from build123d import *

# Parameters (mm, degrees)
F0_W         = 69
F0_H         = 5.7454954955
F1_DEPTH     = 2050
F2_W         = 10
F2_H         = 101.5
F3_DEPTH     = 7.5
F7_DEPTH     = 84
F10_DEPTH    = 90
F11_T1_DEPTH = 134.5
F12_T1_DEPTH = 139.5


# Not quite as in the source:
# - a fillet or chamfer that OpenCascade refuses, or shapes differently, is made with other operations: its cross-section is extruded or revolved along the edge and cut away or added


with BuildPart() as f1:
    # F0 (on Right) → F1 (new body)
    with BuildSketch(Plane.YZ):
        with BuildLine():
            ThreePointArc((-53.5, -33.75), (-51.1568542495, -39.4068542495), (-45.5, -41.75))
            Line((-45.5, -41.75), (0, -41.75))
            Line((0, -41.75), (0, -36.0045045045))
            Line((0, -36.0045045045), (-45.5, -36.0045045045))
            ThreePointArc((-45.5, -36.0045045045), (-48.3284271247, -34.8329316293), (-49.5, -32.0045045045))
            Line((-49.5, -32.0045045045), (-49.5, 32.0045045045))
            ThreePointArc((-49.5, 32.0045045045), (-48.3284271247, 34.8329316293), (-45.5, 36.0045045045))
            Line((-45.5, 36.0045045045), (0, 36.0045045045))
            Line((0, 36.0045045045), (0, 41.75))
            Line((0, 41.75), (-45.5, 41.75))
            ThreePointArc((-45.5, 41.75), (-51.1568542495, 39.4068542495), (-53.5, 33.75))
            Line((-53.5, 33.75), (-53.5, -33.75))
        make_face()
        with Locations((34.5, 38.8772522523)):
            Rectangle(F0_W, F0_H)
        with Locations((34.5, -38.8772522523)):
            Rectangle(F0_W, F0_H)
    extrude(amount=-F1_DEPTH)

    # F2 (on face) → F3 (join)
    with BuildSketch(Plane.XY.offset(41.75)):
        with Locations((-2039, 8.25)):
            Rectangle(F2_W, F2_H)
    extrude(amount=F3_DEPTH)

    # F5: F1 across plane


with BuildPart() as f1_1:
    add(f1.part)
    add(f1.part.mirror(Plane.YZ.offset(-1025)))

    # F6 (on face) → F7 (cut)
    with BuildSketch(Plane.XY.offset(41.75)):
        with BuildLine():
            Line((-2001, 39.5), (-2001, 0))
            Line((-2001, 0), (-2001, -37.5))
            ThreePointArc((-2001, -37.5), (-1998.6568542495, -43.1568542495), (-1993, -45.5))
            Line((-1993, -45.5), (-1925.5, -45.5))
            Line((-1925.5, -45.5), (-1925.5, -41.25))
            Line((-1925.5, -41.25), (-1984.9698543549, -41.25))
            Line((-1984.9698543549, -41.25), (-1992.75, -41.25))
            ThreePointArc((-1992.75, -41.25), (-1995.5784271247, -40.0784271247), (-1996.75, -37.25))
            Line((-1996.75, -37.25), (-1996.75, 0))
            Line((-1996.75, 0), (-1996.75, 39.25))
            ThreePointArc((-1996.75, 39.25), (-1995.5784271247, 42.0784271247), (-1992.75, 43.25))
            Line((-1992.75, 43.25), (-1925.5, 43.25))
            Line((-1925.5, 43.25), (-1925.5, 47.5))
            Line((-1925.5, 47.5), (-1993, 47.5))
            ThreePointArc((-1993, 47.5), (-1998.6568542495, 45.1568542495), (-2001, 39.5))
        make_face()
    extrude(amount=-F7_DEPTH, mode=Mode.SUBTRACT)

    # F8: F1 across plane


with BuildPart() as f1_2:
    add(f1_1.part)
    add(f1_1.part.mirror(Plane.YZ.offset(-1025)), mode=Mode.INTERSECT)

    # F9 (on face) → F10 (cut)
    with BuildSketch(Plane.XY.offset(41.75)):
        with BuildLine():
            ThreePointArc((-1024.0666470126, -40.75), (-1021.1231056256, -43.8556546004), (-1017, -45))
            Line((-1017, -45), (-950, -45))
            Line((-950, -45), (-950, -40.75))
            Line((-950, -40.75), (-1016.75, -40.75))
            ThreePointArc((-1016.75, -40.75), (-1019.5784271247, -39.5784271247), (-1020.75, -36.75))
            Line((-1020.75, -36.75), (-1020.75, 1.25))
            Line((-1020.75, 1.25), (-1020.75, 39.25))
            ThreePointArc((-1020.75, 39.25), (-1019.5784271247, 42.0784271247), (-1016.75, 43.25))
            Line((-1016.75, 43.25), (-950, 43.25))
            Line((-950, 43.25), (-950, 47.5))
            Line((-950, 47.5), (-1017, 47.5))
            ThreePointArc((-1017, 47.5), (-1021.1231056256, 46.3556546004), (-1024.0666470126, 43.25))
            Line((-1024.0666470126, 43.25), (-1025.9333529874, 43.25))
            ThreePointArc((-1025.9333529874, 43.25), (-1028.8768943744, 46.3556546004), (-1033, 47.5))
            Line((-1033, 47.5), (-1100, 47.5))
            Line((-1100, 47.5), (-1100, 43.25))
            Line((-1100, 43.25), (-1033.25, 43.25))
            ThreePointArc((-1033.25, 43.25), (-1030.4215728753, 42.0784271247), (-1029.25, 39.25))
            Line((-1029.25, 39.25), (-1029.25, 1.25))
            Line((-1029.25, 1.25), (-1029.25, -36.75))
            ThreePointArc((-1029.25, -36.75), (-1030.4215728753, -39.5784271247), (-1033.25, -40.75))
            Line((-1033.25, -40.75), (-1100, -40.75))
            Line((-1100, -40.75), (-1100, -45))
            Line((-1100, -45), (-1033, -45))
            ThreePointArc((-1033, -45), (-1028.8768943744, -43.8556546004), (-1025.9333529874, -40.75))
            Line((-1025.9333529874, -40.75), (-1024.0666470126, -40.75))
        make_face()
    extrude(amount=-F10_DEPTH, mode=Mode.SUBTRACT)

    # F11: fillet of radius 4 on 1 edges, made by hand

    # F11_s2 → F11_t1 (cut)
    with BuildSketch(Plane.XZ.offset(-79)):
        with BuildLine():
            ThreePointArc((-2046, -41.75), (-2048.8284271247, -40.5784271247), (-2050, -37.75))
            Line((-2050, -37.75), (-2050, -41.75))
            Line((-2050, -41.75), (-2046, -41.75))
        make_face()
    extrude(amount=F11_T1_DEPTH, mode=Mode.SUBTRACT)

    # F12: fillet of radius 5 on 1 edges, made by hand

    # F12_s2 → F12_t1 (cut)
    with BuildSketch(Plane.XZ.offset(-81.5)):
        with BuildLine():
            ThreePointArc((0, -36.75), (-1.4644660941, -40.2855339059), (-5, -41.75))
            Line((-5, -41.75), (0, -41.75))
            Line((0, -41.75), (0, -36.75))
        make_face()
    extrude(amount=F12_T1_DEPTH, mode=Mode.SUBTRACT)


solid = f1_2.part
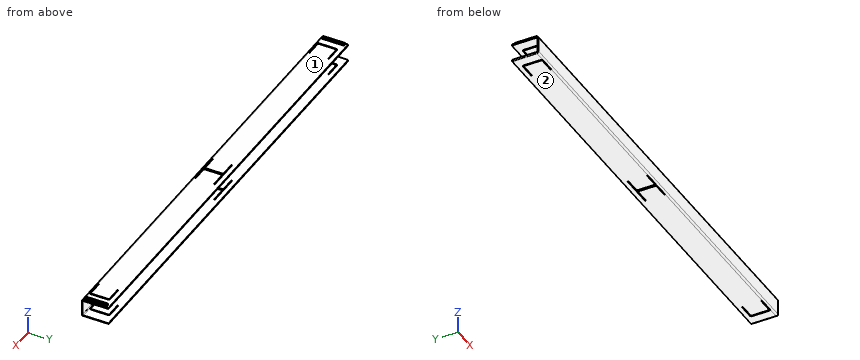
Source: CAD feature listing. Evaluate the final solid. Frame: model axes, mm. Face numbers are marked on the shaded views. Round coordinates to 2 decimals unless told otherwise and drop trailing zeros. Order: outer loops, then holes, each group sorted by start corner. A loop starts at its lowest first (then second) coordinate and runs counter-clockwise, first axis right, second up. Notation, with made-up numbers: (-2.5, 46) -> (29.5, 46) arc R9 cw to (29.5, 63) -> close; hole circle Ø8 at (74, -24). An arc over 180 degrees is marked (long way). Answer as CSV lines item,"result".
Item 1: Section C-C, the plane y = 2. Count the separate pieces of the cut face and the enclosed holes in it, plus the area to 3 significant figures.
A:
separate pieces,"8"
enclosed holes,"0"
area,"23,500 mm²"
Item 2: Section B-B, the plane z = 13. Return loops of the section in (x, y), plus the area to 3 significant figures.
A:
outline,"(-2050, -53.5) -> (0, -53.5) -> (0, -49.5) -> (-2050, -49.5) -> close"
area,"8,200 mm²"
Item 3: Section A-A, the plane x = -471. Return loops of the section in (y, z), plus the area to 3 significant figures.
A:
outline,"(-53.5, -33.75) arc R8 ccw to (-45.5, -41.75) -> (69, -41.75) -> (69, -36) -> (-45.5, -36) arc R4 cw to (-49.5, -32) -> (-49.5, 32) arc R4 cw to (-45.5, 36) -> (69, 36) -> (69, 41.75) -> (-45.5, 41.75) arc R8 ccw to (-53.5, 33.75) -> close"
area,"1,680 mm²"
Item 4: Pin query (flat end, axial travel): pin 1 Ø3 at (x, z) = (-106, 38.5) entering from -Y; pin 2 Ø2 at (x, z) = (-2038.5, 47) entering from +Y; pin 3 Ø2 at (x, y) = (-1413, 16.5) entering from +Z. Return the tip coordinate at first contact, or that it passes through.
A:
pin 1,"y = -52.81"
pin 2,"y = 59"
pin 3,"z = 41.75"
Item 5: Pull-direction query (X, two-part tool) for the marked faces 1 and 2; classes: pulls with the +X half, pulls with the -X half, needs draft (parallel to the pull), parting line crosses it, or undercut.
A:
face 1,"undercut"
face 2,"needs draft"
Item 6: Line query: L1, parallel to Z at x = -637, y = 64; L2, parallel to Y at x = -201.5, z = 26.5; L3, parallel to Y at x = -332, z = 34. Output: solid intervals per line, ascending.
A:
L1,"-41.75 to -36, 36 to 41.75"
L2,"-53.5 to -49.5"
L3,"-53.5 to -48.97"
